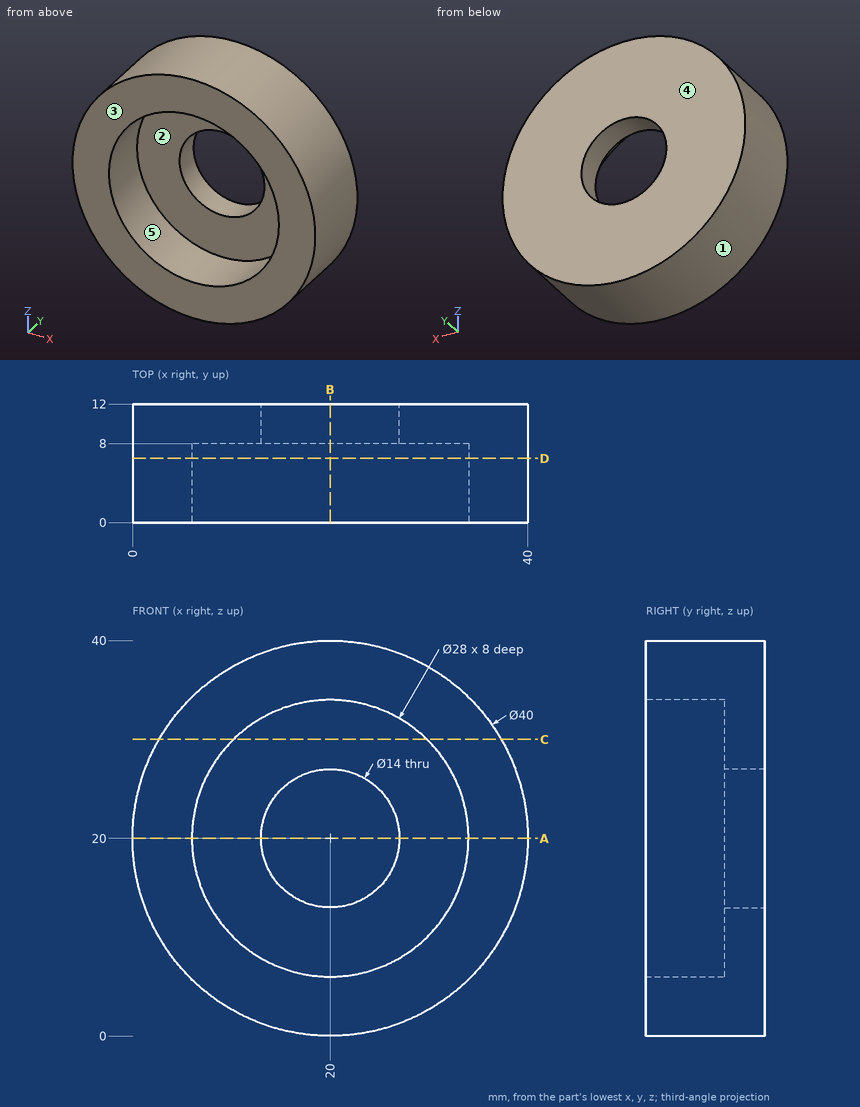
Source: three-view drawing plus pictorial views. Frame: mm from the lowest corner of the part. A direction names the side the tool comes from. Coordinates: 2 decimals unless noted, no trailing zeros. Loops run counter-clockwise (first coordinate to the right, second up) from the corner with the lowest first, then second, coordinate; pieces in that order, holes last. Notation, with made-up numbers: (88, 51.25) -> (125, 51.25) arc R32 ccw to (125, 86.25) -> close; hole circle Ø8 at (-30.75, 3.25). An arc over 180 degrees is marked (long way). Answer in a Markdown table with one row per item. Add a question column.
Q1. Section D-D on y = 6.5. Return the cut outline in (x, z).
Q2. Ray query, line 1 along X through (y, z) = (9.85, 20); line 2 along X through (y, z) = (4.5, 20); line 3 along Y through (x, z) = (29, 21.5). Return the intervals inside material, ascending.
Q3. Section B-B on x = 20. Return the cut outline in (y, z), and give its area (3 significant figures).
Q4. Contact query for flat-ended pins moving along their axis: pin 1 Ø22.5 at (x, z) = (23.5, 23) entering from -Y; pin 2 Ø1.5 at (x, z) = (28.5, 21) entering from -Y; pin 3 Ø2 at (x, y) = (14, 5) entering from -Z; pin 4 Ø5 at (x, y) = (35.5, 3) entering from -Z. Output: stop coordinate, or through.
Q5. Reachability of the marked faces 4 and 5 from +Z, -Z, +X, -X, +Y, -Y: full face, straight path, thin tool, end or side. Return the list, or none.
Q6. Pull-direction query (Z, two-part tool) for the marked faces 1, 2 and 3; classes: pulls with the +Z half, pulls with the -Z half, needs draft (parallel to the pull), parting line crosses it, or undercut.
Q7. Section A-A on z = 20. Return the cut outline in (x, y).
Q8. Section C-C on z = 30. Return the cut outline in (x, y).
Computed values:
| question | item | result |
|---|---|---|
| 1 | outline | circle Ø40 at (20, 20); hole circle Ø28 at (20, 20) |
| 2 | line 1 | x = 0 to 13, 27 to 40 |
| 2 | line 2 | x = 0 to 6, 34 to 40 |
| 2 | line 3 | y = 8 to 12 |
| 3 | outline | (0, 0) -> (12, 0) -> (12, 13) -> (8, 13) -> (8, 6) -> (0, 6) -> close; (0, 34) -> (8, 34) -> (8, 27) -> (12, 27) -> (12, 40) -> (0, 40) -> close |
| 3 | area | 200 mm^2 |
| 4 | pin 1 | stops at y = 0 |
| 4 | pin 2 | stops at y = 8 |
| 4 | pin 3 | stops at z = 0.64 |
| 4 | pin 4 | stops at z = 4.8 |
| 5 | face 4 | +Z, -Z, +X, -X, +Y |
| 5 | face 5 | -Y |
| 6 | face 1 | parting line crosses it |
| 6 | face 2 | undercut |
| 6 | face 3 | needs draft |
| 7 | outline | (0, 0) -> (6, 0) -> (6, 8) -> (13, 8) -> (13, 12) -> (0, 12) -> close; (27, 8) -> (34, 8) -> (34, 0) -> (40, 0) -> (40, 12) -> (27, 12) -> close |
| 8 | outline | (2.68, 0) -> (10.2, 0) -> (10.2, 8) -> (29.8, 8) -> (29.8, 0) -> (37.32, 0) -> (37.32, 12) -> (2.68, 12) -> close |
